Autodesk Inventor part; units mm, degrees
ref_plane "YZ Plane" through (0, 0, 0) normal (1, 0, 0) x (0, 1, 0)
ref_plane "XZ Plane" through (0, 0, 0) normal (0, 1, 0) x (-1, 0, 0)
ref_plane "XY Plane" through (0, 0, 0) normal (0, 0, 1) x (1, 0, 0)
sketch "Sketch1" plane through (0, 0, 0) normal (1, 0, 0) x (0, 1, 0)
  line L0 (0, 0) -> (127, 0)
  line L1 (127, 0) -> (127, 50.8)
  line L2 (0, 0) -> (0, 50.8)
  arc A0 (95.25, 82.55) -> (127, 50.8) centre (95.25, 50.8) ccw construction
  arc A1 (31.75, 82.55) -> (0, 50.8) centre (31.75, 50.8) ccw
  line L3 (95.25, 82.55) -> (31.75, 82.55)
  arc A2 (127, 50.8) -> (95.25, 82.55) centre (95.25, 50.8) ccw
  line L4 (127, 19.05) -> (0, 19.05) construction
  dimension "d0" = 127
  dimension "d1" = 63.5
  dimension "d2" = 19.05
extrude "Extrusion1" add sketch "Sketch1" along normal blind 990.6
fillet "Fillet1" radius 31.75 10 edges at (990.6, 0, 25.4) (990.6, 63.5, 82.55) (990.6, 117.7006, 73.2506) (990.6, 127, 25.4) (990.6, 9.2994, 73.2506) (0, 0, 25.4) (0, 63.5, 82.55) (0, 117.7006, 73.2506) (0, 127, 25.4) (0, 9.2994, 73.2506)
properties part number "Back Bumper"
Geometry check sheet. Reference: the model listing, model coordinates, mm. Coordinates: 2 decimals unless noted, no trailing zeros. Write each loop counter-clockwise with the first axis right and the second up, starting at its lowest first coordinate (ties: lowest second). Pieces come first, ordered by that corner, then holes. Notation, with made-up numbers: M 16,6.5 L 64,6.5 A19 cw 64,30.5 Z; hole C 87,18.5 d10. An arc over 180 degrees is marked long. Use one line per item in the form item = value. Start each with the question number.
1) Thickness scan on probe 1 along X at (y, z) = (98, 28.5); probe 2 along Y at (x, z) = (674.5, 53); probe 3 along X at (y, z) = (28.5, 15.5). Record the ranges inside material, lowest first. Write a range as from..to.
2) Section check A-A on x = 260.5. Enter the section's corners in (y, z).
3) Go/stop test with flat-tipped pins: pin 1 Ø2 at (x, z) = (819, 34.5) entering from -Y; pin 2 Ø6 at (x, y) = (357, 112.5) entering from +Z; pin 3 Ø8 at (x, z) = (852, 69.5) entering from +Y; pin 4 Ø1.5 at (x, z) = (766.5, 60) entering from -Y. Record where each tip stops, or that it passes through.
4) Section check B-B on z = 66. Enter the section's corners in (x, y), and give its area (3 significant figures).
Responses:
q1.probe_1 = 0.12..990.48
q1.probe_2 = 0.08..126.92
q1.probe_3 = 0.17..990.43
q2.outline = M 0,0 L 127,0 L 127,50.8 A31.75 ccw 95.25,82.55 L 31.75,82.55 A31.75 ccw 0,50.8 Z
q3.pin_1 = 0
q3.pin_2 = 79.17
q3.pin_3 = 123.39
q3.pin_4 = 1.15
q4.outline = M 3.87,31.75 A27.88 ccw 31.75,3.87 L 958.85,3.87 A27.88 ccw 986.73,31.75 L 986.73,95.25 A27.88 ccw 958.85,123.13 L 31.75,123.13 A27.88 ccw 3.87,95.25 Z
q4.area = 117,000 mm2
